Check sheet for the drawn part. Datum: minimum x, y, z corner. Units: mm. A direction names the side the tool comes from. Coordinates: 2 decimals unless noted, no trailing zeros. Loops run counter-clockwise (first coordinate to the right, second up) from the corner with the lowest first, then second, coordinate; pieces in that order, holes last. Notation, with made-up numbers: (-23, -24) - (-14, -24) arc R21 cw to (-14, 14) - close; hole circle Ø6 at (47.5, 63.5). An arc over 180 degrees is marked (long way). Answer as a JSON object with one key per item and string values. Group by question number.
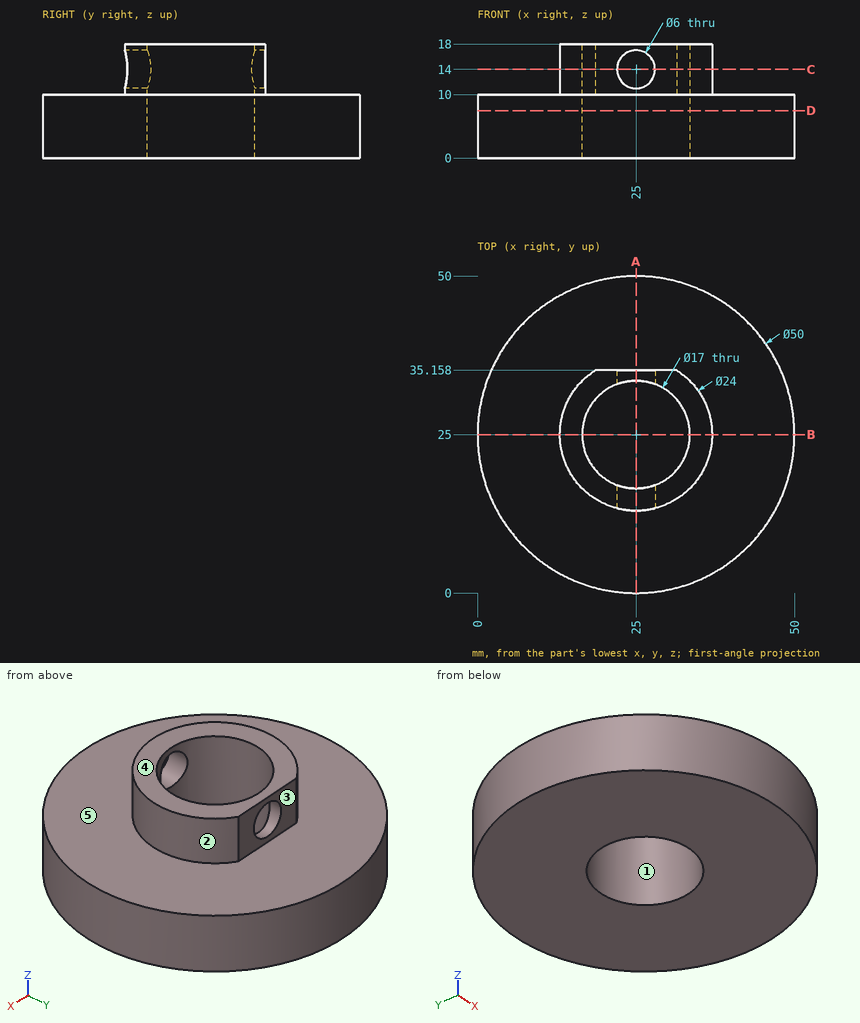
1. Sectioned sample at D-D on z = 7.5. Record the cut outline in (x, y).
2. Sectioned sample at A-A on x = 25. Record the cut outline in (y, z).
3. Access from +Z, -Z, +X, -X, +Y, -Y to the whole of each face (thin tool, end or side, straight path). Record for the marked faces 4 and 5.
4. Sectioned sample at C-C on z = 14. Record the cut outline in (x, y).
5. Release check for a two-part mould opening along Y. For the marked faces 1, 2 and 3 record: released by +Y, released by -Y, zero draft, split by the parting line, or undercut.
6. Sectioned sample at B-B on y = 25. Record the cut outline in (x, z).
7. Gauge pin test, flat ends, axial feed: pin 1 (2 mm diameter, centred on x = 37, z = 14, fed in from -Y) (1 decimal); pin 2 (3 mm diameter, centred on x = 38.5, y = 10, fed in from +Z); pin 3 (6 mm diameter, centred on x = 13, z = 6, fed in from -Y). Record the tip position at first contact, or that the pin passes through.
8. Material ranges on line 1 (Z direction, x = 25, y = 34.4); line 2 (Y direction, x = 25, z = 5.25); line 3 (Z direction, x = 26.5, y = 44.5), recorded low to high.
Answers follow:
{
 "1": {"outline": "circle Ø50 at (25, 25); hole circle Ø17 at (25, 25)"},
 "2": {"outline": "(0, 0) - (16.5, 0) - (16.5, 11) - (13, 11) - (13, 10) - (0, 10) - close; (13, 17) - (16.5, 17) - (16.5, 18) - (13, 18) - close; (33.5, 0) - (50, 0) - (50, 10) - (35.16, 10) - (35.16, 11) - (33.5, 11) - close; (33.5, 17) - (35.16, 17) - (35.16, 18) - (33.5, 18) - close"},
 "3": {"face 4": "+Z, +X, -X, +Y, -Y", "face 5": "+Z"},
 "4": {"outline": "(18.61, 35.16) arc R12 ccw to (22, 13.38) - (22, 17.05) arc R8.5 cw to (22, 32.95) - (22, 35.16) - close; (28, 13.38) arc R12 ccw to (31.39, 35.16) - (28, 35.16) - (28, 32.95) arc R8.5 cw to (28, 17.05) - close"},
 "5": {"face 1": "undercut", "face 2": "split by the parting line", "face 3": "released by +Y"},
 "6": {"outline": "(0, 0) - (16.5, 0) - (16.5, 18) - (13, 18) - (13, 10) - (0, 10) - close; (33.5, 0) - (50, 0) - (50, 10) - (37, 10) - (37, 18) - (33.5, 18) - close"},
 "7": {"pin 1": "stops at y = 20.2", "pin 2": "stops at z = 10", "pin 3": "stops at y = 1.68"},
 "8": {"line 1": "z = 0 to 11, 17 to 18", "line 2": "y = 0 to 16.5, 33.5 to 50", "line 3": "z = 0 to 10"}
}
